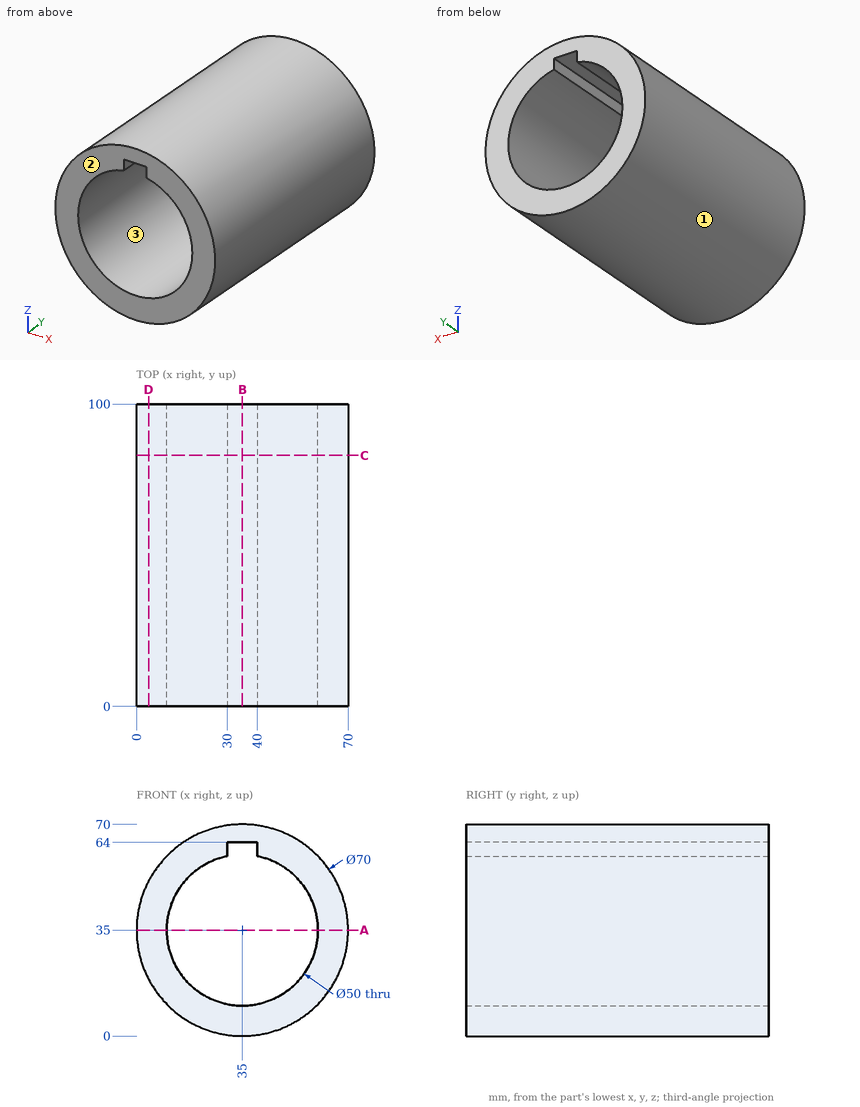
Can you work these out from the drawing? Everything is in mm from the part's minimum corner. Give positions to 0.01 mm unless a question says otherwise; leave off trailing zeros. Order: outer loops, then holes, each group sorted by start corner. A loop starts at its lowest first (then second) coordinate and runs counter-clockwise, first axis right, second up. Notation, with made-up numbers: M 72.25,45 L 94.25,45 A5 cw 94.25,49 Z; hole C -19.75,-21.5 d9. An arc over 180 degrees is marked long. One line per question, with ' | ' between items.
1. I want a section at D-D (x = 4). List the corners of the cut face in (y, z) for me.
Results:
outline: M 0,18.75 L 100,18.75 L 100,51.25 L 0,51.25 Z
2. We'd pull the mould along X, two halves only. Please class the marked faces 1, 2 and 3: +X half, -X half, draft (parallel to the pull), parting line (faces both ways), or undercut.
Results:
face 1: parting line | face 2: draft | face 3: undercut
3. I want a section at C-C (y = 83). List the corners of the cut face in (x, z) for me.
Results:
outline: C 35,35 d70; hole M 30,59.49 A25 ccw long 40,59.49 L 40,64 L 30,64 Z
4. I want a section at A-A (z = 35). List the corners of the cut face in (x, y) for me.
Results:
outline: M 0,0 L 10,0 L 10,100 L 0,100 Z; M 60,0 L 70,0 L 70,100 L 60,100 Z
5. If I drill on line 1 (Z direction, x = 35, y = 55); line 2 (Z direction, x = 37, y = 70); line 3 (X direction, y = 8, z = 12), over which ranges is the centre line in solid material (lowest first)?
Results:
line 1: 0 to 10, 64 to 70 | line 2: 0.06 to 10.08, 64 to 69.94 | line 3: 8.62 to 25.2, 44.8 to 61.38
6. I want a section at B-B (x = 35). List the corners of the cut face in (y, z) for me, and give its area (3 significant figures).
Results:
outline: M 0,0 L 100,0 L 100,10 L 0,10 Z; M 0,64 L 100,64 L 100,70 L 0,70 Z | area: 1,600 mm²
7. I'm going to push flat-ended pins straight in: pin 1 (5 mm diameter, centred on y = 69, z = 61.5, fed in from +X); pin 2 (6 mm diameter, centred on y = 30, z = 62.5, fed in from -X) (3 decimals); pin 3 (3 mm diameter, centred on x = 33, y = 39, fed in from -Z). Where does each tip first touch, or does it pass through?
Results:
pin 1: x = 60.48 | pin 2: x = 10.005 | pin 3: z = 0
